from build123d import *

# Parameters (mm, degrees)
F0_R          = 25
F1_DEPTH      = 50
F2_SIZE       = 5
F3_R          = 7
F4_DEPTH      = 80
F4_DEPTH_BACK = 25
F3_R_2        = 10
F5_DEPTH      = 2
F6_START      = -12
F6_DEPTH      = 8


with BuildPart() as f1:
    # F0 (on Front) → F1 (new body, symmetric)
    with BuildSketch(Plane.XZ):
        with BuildLine():
            ThreePointArc((-45.5384452963, 12.5), (-41.0059538996, 10.4314783147), (-39.5986480837, 5.652173913))
            ThreePointArc((-39.5986480837, 5.652173913), (-40, 0), (-39.5986480837, -5.652173913))
            ThreePointArc((-39.5986480837, -5.652173913), (-41.0059538996, -10.4314783147), (-45.5384452963, -12.5))
            Line((-45.5384452963, -12.5), (-66.0473750966, -12.5))
            ThreePointArc((-66.0473750966, -12.5), (-68.1686954401, -13.3786796564), (-69.0473750966, -15.5))
            Line((-69.0473750966, -15.5), (-69.0473750966, -24.5))
            ThreePointArc((-69.0473750966, -24.5), (-68.1686954401, -26.6213203436), (-66.0473750966, -27.5))
            Line((-66.0473750966, -27.5), (-34.9106001094, -27.5))
            ThreePointArc((-34.9106001094, -27.5), (-29.8541011409, -28.3779669246), (-25.3895273523, -30.9090909091))
            ThreePointArc((-25.3895273523, -30.9090909091), (40, 0), (-25.3895273523, 30.9090909091))
            ThreePointArc((-25.3895273523, 30.9090909091), (-29.8541011409, 28.3779669246), (-34.9106001094, 27.5))
            Line((-34.9106001094, 27.5), (-66.0473750966, 27.5))
            ThreePointArc((-66.0473750966, 27.5), (-68.1686954401, 26.6213203436), (-69.0473750966, 24.5))
            Line((-69.0473750966, 24.5), (-69.0473750966, 15.5))
            ThreePointArc((-69.0473750966, 15.5), (-68.1686954401, 13.3786796564), (-66.0473750966, 12.5))
            Line((-66.0473750966, 12.5), (-45.5384452963, 12.5))
        make_face()
        Circle(F0_R, mode=Mode.SUBTRACT)
    extrude(amount=F1_DEPTH, both=True)

    # F2
    f2_edges = [f1.edges().sort_by_distance(p)[0] for p in [
        (-25, -50, 0),
        (-25, 50, 0),
    ]]
    chamfer(f2_edges, length=F2_SIZE)

    # F3 (on face) → F4 (cut, two sides)
    with BuildSketch(Plane.XY.offset(27.5)) as f4_sk:
        with Locations((-50, 0)):
            Circle(F3_R)
    extrude(amount=-F4_DEPTH, mode=Mode.SUBTRACT)
    extrude(f4_sk.sketch, amount=F4_DEPTH_BACK, mode=Mode.SUBTRACT)

    # F3 (on face) → F5 (cut)
    with BuildSketch(Plane.XY.offset(27.5)):
        with Locations((-50, 0)):
            Circle(F3_R_2)
        with Locations((-50, 0)):
            Circle(F3_R, mode=Mode.SUBTRACT)
    extrude(amount=-F5_DEPTH, mode=Mode.SUBTRACT)

    # F3 (on face) → F6 (cut)
    with BuildSketch(Plane.XY.offset(27.5).offset(F6_START)):
        with Locations((-50, 0)):
            Circle(F3_R_2)
        with Locations((-50, 0)):
            Circle(F3_R, mode=Mode.SUBTRACT)
    extrude(amount=-F6_DEPTH, mode=Mode.SUBTRACT)


solid = f1.part
The model under review builds one solid part; all positions refer to its coordinate system, in mm. A direction names the side the tool comes from. Coordinates: 2 decimals unless noted, no trailing zeros. Write each loop counter-clockwise with the first axis right and the second up, starting at its lowest first coordinate (ties: lowest second). Pieces come first, ordered by that corner, then holes. Notation, with made-up numbers: (-27, 58) - (-16, 58) arc R17 ccw to (-16, 82) - close; hole circle Ø3 at (51.5, -5). An arc over 180 degrees is marked (long way). Answer as a JSON object with one key per item and string values. Group by question number.
1. Machinability: for faces 1 (the face through (-61, -1, 27.5)), 2 (the face through (-60, 0, 27)), 3 (the face through (-68.15, -0.7, -13.36)), 4 (the face through (-40.46, 3, 13.69)), which of the approach directions +Z, -Z, +X, -X, +Y, -Y give a long, thin tool a straight path to every point of the face, cutting with its end or side? Answer none if there is none.
2. To check wall thickness, follow probe 1 along Z at (x, y) = (-55.5, 20); probe 2 along Y at (x, z) = (-50, 13); probe 3 along Z at (x, y) = (2, 38). State the ranges of each line that lie inside material, in increasing order.
3. Add section C-C (x = -50). Give the boundary of the cut face in (y, z).
4. Mouldability with a two-part tool opening along Z and no side actions: class faces 5 (the face through (-43.323, 2.103, -19.609)), 6 (the face through (-40.96, -0.7, -10.38)), 7 (the face through (-68.15, -0.7, 26.64)) as pulls with the +Z half, pulls with the -Z half, needs draft (parallel to the pull), parting line crosses it, or undercut.
5. Add section D-D (x = 0). Give the boundary of the cut face in (y, z), plus the area to 3 significant figures.
6. Add section B-B (z = 0). Give the boundary of the cut face in (x, y), plus the area to 3 significant figures.
7. Add section A-A (y = 0). Give the number of separate pieces and of enclosed holes in the cut face, plus the area to 3 significant figures.
8. Clearance check with flat-ended pins moving along their axes: pin 1 Ø9.5 at (x, y) = (-43.5, 20) entering from -Z; pin 2 Ø6 at (x, y) = (-30.5, 32.5) entering from -Z; pin 3 Ø3 at (y, z) = (14.5, -13) entering from +X; pin 4 Ø12.5 at (x, y) = (-50, 0) entering from +Z. State where each tip first meets the part, or that it passes through.
Findings:
{
 "1": {"face 1": "+Z, -X, +Y, -Y", "face 2": "+Z", "face 3": "-X, +Y, -Y", "face 4": "none"},
 "2": {"probe 1": "-27.5 to -12.5, 12.5 to 27.5", "probe 2": "-50 to -10, 10 to 50", "probe 3": "-39.95 to -24.92, 24.92 to 39.95"},
 "3": {"outline": "(-50, -27.5) - (-7, -27.5) - (-7, -12.5) - (-50, -12.5) - close; (-50, 12.5) - (-10, 12.5) - (-10, 15.5) - (-7, 15.5) - (-7, 25.5) - (-10, 25.5) - (-10, 27.5) - (-50, 27.5) - close; (7, -27.5) - (50, -27.5) - (50, -12.5) - (7, -12.5) - close; (7, 15.5) - (10, 15.5) - (10, 12.5) - (50, 12.5) - (50, 27.5) - (10, 27.5) - (10, 25.5) - (7, 25.5) - close"},
 "4": {"face 5": "needs draft", "face 6": "undercut", "face 7": "pulls with the +Z half"},
 "5": {"outline": "(-50, -40) - (50, -40) - (50, -30) - (45, -25) - (-45, -25) - (-50, -30) - close; (-50, 30) - (-45, 25) - (45, 25) - (50, 30) - (50, 40) - (-50, 40) - close", "area": "2,950 mm²"},
 "6": {"outline": "(-40, -50) - (-30, -50) - (-25, -45) - (-25, 45) - (-30, 50) - (-40, 50) - close; (25, -45) - (30, -50) - (40, -50) - (40, 50) - (30, 50) - (25, 45) - close", "area": "2,950 mm²"},
 "7": {"separate pieces": "3", "enclosed holes": "1", "area": "3,670 mm²"},
 "8": {"pin 1": "z = -27.5", "pin 2": "z = -29.46", "pin 3": "x = 38.31", "pin 4": "through"}
}
